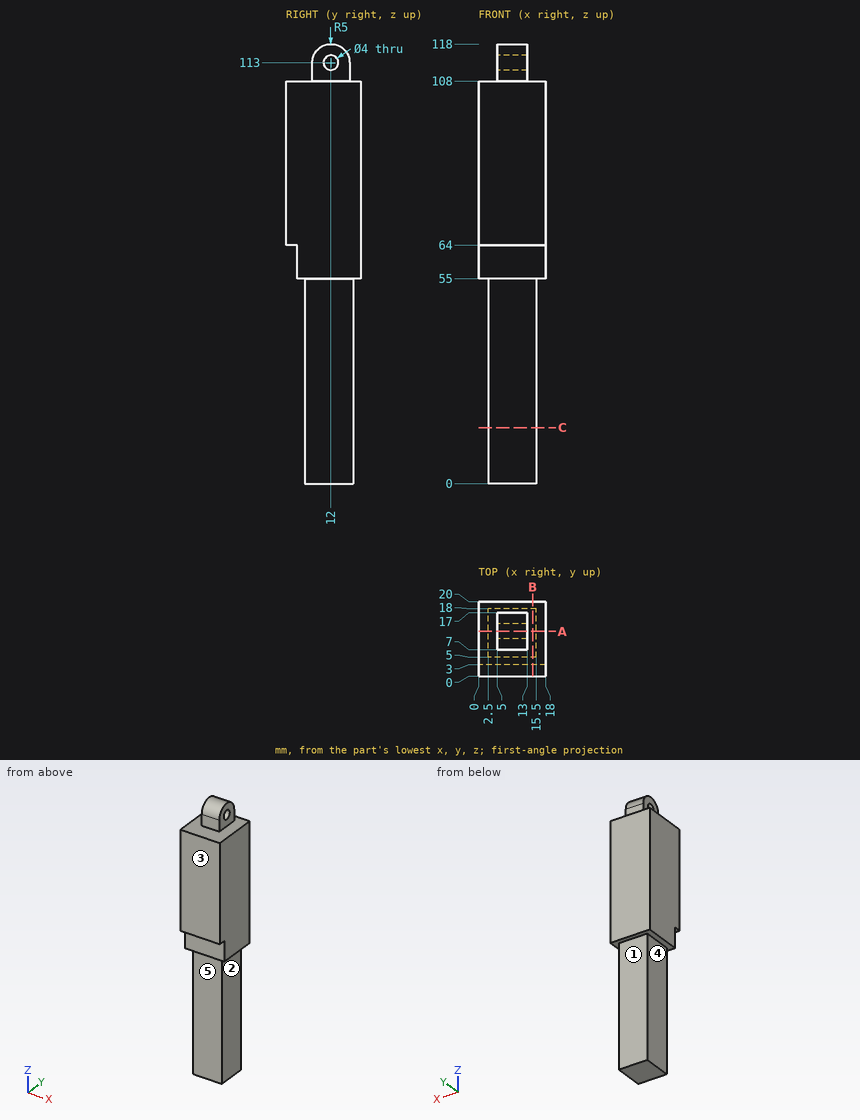
Here's the drawing with two shaded views (mm, measured from the low corner). I have some questions. A direction names the side the tool comes from. Round coordinates to 2 decimals unless told otherwise and drop trailing zeros. Order: outer loops, then holes, each group sorted by start corner. A loop starts at its lowest first (then second) coordinate and runs counter-clockwise, first axis right, second up. Notation, with made-up numbers: M 75,-16 L 120,-16 A25 cw 120,21 Z; hole C 59.5,23 d10. An arc over 180 degrees is marked long. Use CSV: the item, a comma, the result in double quotes.
1) I want a section at A-A (y = 12). List the corners of the cut face in (x, z) for me.
Taken from the geometry:
outline,"M 0,55 L 2.5,55 L 2.5,0 L 15.5,0 L 15.5,55 L 18,55 L 18,108 L 13,108 L 13,111 L 5,111 L 5,108 L 0,108 Z; M 5,115 L 13,115 L 13,118 L 5,118 Z"
2) On a 3-axis mill with a long thin cutter (end or side, diameter ignored), from which of +Z, -Z, +X, -X, +Y, -Y can I reach the whole of each face in a straight line? I mean the marked faces 1, 2, 3, 4 and 5. Say none if no direction works.
Taken from the geometry:
face 1,"-Z, +X, -X, +Y"
face 2,"-Z, +X, +Y, -Y"
face 3,"+Z, -Z, +X, -X, -Y"
face 4,"-Z, -X, +Y, -Y"
face 5,"-Z, +X, -X, -Y"
3) I need wall thicknesses on line 1 along Y through (x, z) = (8, 113); line 2 along X through (y, z) = (12.5, 35.5); line 3 along Y through (x, z) = (8, 51). Which ranges of each line are inside material? Lowest first, please. Write a range as [from, to].
Taken from the geometry:
line 1,"[7, 10], [14, 17]"
line 2,"[2.5, 15.5]"
line 3,"[5, 18]"
4) I'm going to push flat-ended pins straight in: P1, Ø1.5, axis at x = 3, y = 7, coming from the +Z side; P2, Ø4, axis at x = 14.5, y = 11, coming from the -Z side; P3, Ø6.5, axis at x = 10, z = 18.5, coming from the -Y side; P4, Ø4, axis at x = 11.5, z = 19.5, coming from the +Y side. Where does each tip first touch, or does it pass through?
Taken from the geometry:
P1,"z = 108"
P2,"z = 0"
P3,"y = 5"
P4,"y = 18"
5) I want a section at B-B (x = 14.5). List the corners of the cut face in (y, z) for me.
Taken from the geometry:
outline,"M 0,64 L 3,64 L 3,55 L 5,55 L 5,0 L 18,0 L 18,55 L 20,55 L 20,108 L 0,108 Z"
6) I want a section at C-C (z = 15). List the corners of the cut face in (x, y) for me.
Taken from the geometry:
outline,"M 2.5,5 L 15.5,5 L 15.5,18 L 2.5,18 Z"
